CAD build for the part. Positions are in the model's coordinates, mm. Round coordinates to 2 decimals unless told otherwise and drop trailing zeros. Write each loop counter-clockwise with the first axis right and the second up, starting at its lowest first coordinate (ties: lowest second). Pieces come first, ordered by that corner, then holes. Notation, with made-up numbers: (-0.75, 43.5) - (18.25, 43.5) arc R15 cw to (18.25, 47.5) - close; hole circle Ø3 at (-20, 4.5). An arc over 180 degrees is marked (long way). Put each result on its own line as item: value. Start each with the question number.
Item 1: Cut at C-C (z = 3). Give the cut face in (x, y).
Item 2: Drill centre lines: line 1 (Z direction, x = 18, y = 3.9); line 2 (X direction, y = 1.05, z = 0); line 3 (X direction, y = 0.4, z = -0.75). Where is each one in solid material? Low to high. Write a range as from..to.
Item 3: Cut at B-B (y = 2.85). Count the separate pieces of the cut face and the enclosed holes in it, and give its area (3 significant figures).
Item 4: Cut at A-A (x = 18.25). Give the cut face in (y, z), and give its area (3 significant figures).
Item 5: Pin check, flat tip, straight feed: pin 1 Ø2 at (y, z) = (3.5, 1) entering from +X. Stop position of the tip, or through.
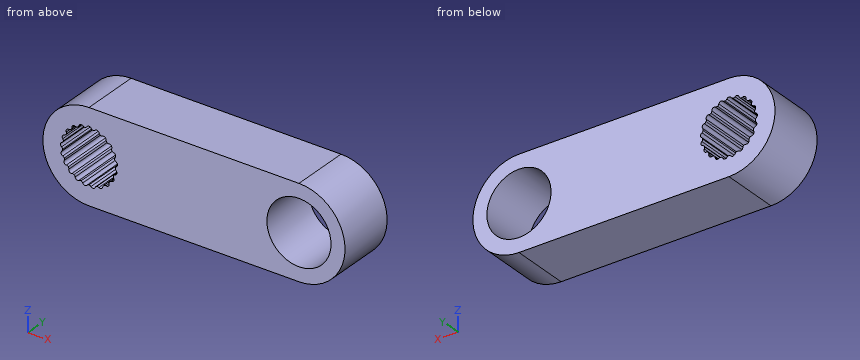
```python
from build123d import *

# Parameters (mm, degrees)
SKETCH1_R           = 3.95
BOSS_EXTRUDE1_DEPTH = 5
BOSS_EXTRUDE2_DEPTH = 5
SKETCH3_R           = 2.75
CUT_EXTRUDE1_DEPTH  = 5


with BuildPart() as part:
    # Sketch1 → Boss-Extrude1 (new body)
    with BuildSketch(Plane(origin=(0, 0, 0), x_dir=(1, 0, 0), z_dir=(0, 1, 0))):
        Circle(SKETCH1_R)
        with BuildLine():
            ThreePointArc((-0.166646614, 2.345141313), (-0.092401566, 2.286261662), (0, 2.2652595))
            ThreePointArc((0, 2.2652595), (0.092401566, 2.286261662), (0.166646614, 2.345141313))
            ThreePointArc((0.166646614, 2.345141313), (0.365153552, 2.422635524), (0.531999564, 2.290073216))
            ThreePointArc((0.531999564, 2.290073216), (0.585591031, 2.211925311), (0.667696959, 2.164620376))
            ThreePointArc((0.667696959, 2.164620376), (0.762183879, 2.157453631), (0.850485509, 2.191833312))
            ThreePointArc((0.850485509, 2.191833312), (1.063015161, 2.207373726), (1.183375246, 2.031522064))
            ThreePointArc((1.183375246, 2.031522064), (1.211551295, 1.941049689), (1.276066113, 1.871645232))
            ThreePointArc((1.276066113, 1.871645232), (1.364242809, 1.836946378), (1.458755034, 1.843771303))
            ThreePointArc((1.458755034, 1.843771303), (1.666423208, 1.795977086), (1.729602845, 1.592461261))
            ThreePointArc((1.729602845, 1.592461261), (1.72985991, 1.497703284), (1.771051193, 1.412366197))
            ThreePointArc((1.771051193, 1.412366197), (1.845082779, 1.353218377), (1.937407773, 1.331882123))
            ThreePointArc((1.937407773, 1.331882123), (2.121762239, 1.225), (2.12214764, 1.011903287))
            ThreePointArc((2.12214764, 1.011903287), (2.094462881, 0.92127937), (2.108670602, 0.827592226))
            ThreePointArc((2.108670602, 0.827592226), (2.161979047, 0.749250985), (2.243913329, 0.701649371))
            ThreePointArc((2.243913329, 0.701649371), (2.388573385, 0.545176288), (2.326130305, 0.341433266))
            ThreePointArc((2.326130305, 0.341433266), (2.272963633, 0.262995741), (2.258925375, 0.169283054))
            ThreePointArc((2.258925375, 0.169283054), (2.286773988, 0.078709355), (2.351037339, 0.009071994))
            ThreePointArc((2.351037339, 0.009071994), (2.443149303, -0.183088729), (2.323426084, -0.3593746))
            ThreePointArc((2.323426084, -0.3593746), (2.249501592, -0.418656214), (2.208464714, -0.504067659))
            ThreePointArc((2.208464714, -0.504067659), (2.208379026, -0.598825947), (2.249261363, -0.68431147))
            ThreePointArc((2.249261363, -0.68431147), (2.280640684, -0.89508551), (2.114275259, -1.028250455))
            ThreePointArc((2.114275259, -1.028250455), (2.026161462, -1.063108727), (1.961772273, -1.13262975))
            ThreePointArc((1.961772273, -1.13262975), (1.933759896, -1.223152935), (1.947628645, -1.316890857))
            ThreePointArc((1.947628645, -1.316890857), (1.915487132, -1.527550015), (1.717261799, -1.605761745))
            ThreePointArc((1.717261799, -1.605761745), (1.622787995, -1.613099364), (1.540767756, -1.660552716))
            ThreePointArc((1.540767756, -1.660552716), (1.487317713, -1.738797417), (1.472940575, -1.832458712))
            ThreePointArc((1.472940575, -1.832458712), (1.380134142, -2.024284997), (1.167662092, -2.040594058))
            ThreePointArc((1.167662092, -2.040594058), (1.075222693, -2.019759044), (0.982859262, -2.040928287))
            ThreePointArc((0.982859262, -2.040928287), (0.908720824, -2.099942118), (0.86737527, -2.185204569))
            ThreePointArc((0.86737527, -2.185204569), (0.722150177, -2.341153374), (0.514310485, -2.294110633))
            ThreePointArc((0.514310485, -2.294110633), (0.432119136, -2.246954269), (0.337619409, -2.239958423))
            ThreePointArc((0.337619409, -2.239958423), (0.249380102, -2.274497747), (0.184739867, -2.343785411))
            ThreePointArc((0.184739867, -2.343785411), (0, -2.45), (-0.184739867, -2.343785411))
            ThreePointArc((-0.184739867, -2.343785411), (-0.249380102, -2.274497747), (-0.337619409, -2.239958423))
            ThreePointArc((-0.337619409, -2.239958423), (-0.432119136, -2.246954269), (-0.514310485, -2.294110633))
            ThreePointArc((-0.514310485, -2.294110633), (-0.722150177, -2.341153374), (-0.86737527, -2.185204569))
            ThreePointArc((-0.86737527, -2.185204569), (-0.908720824, -2.099942118), (-0.982859262, -2.040928287))
            ThreePointArc((-0.982859262, -2.040928287), (-1.075222693, -2.019759044), (-1.167662092, -2.040594058))
            ThreePointArc((-1.167662092, -2.040594058), (-1.380134142, -2.024284997), (-1.472940575, -1.832458712))
            ThreePointArc((-1.472940575, -1.832458712), (-1.487317713, -1.738797417), (-1.540767756, -1.660552716))
            ThreePointArc((-1.540767756, -1.660552716), (-1.622787995, -1.613099364), (-1.717261799, -1.605761745))
            ThreePointArc((-1.717261799, -1.605761745), (-1.915487132, -1.527550015), (-1.947628645, -1.316890857))
            ThreePointArc((-1.947628645, -1.316890857), (-1.933759896, -1.223152935), (-1.961772273, -1.13262975))
            ThreePointArc((-1.961772273, -1.13262975), (-2.026161462, -1.063108727), (-2.114275259, -1.028250455))
            ThreePointArc((-2.114275259, -1.028250455), (-2.280640684, -0.89508551), (-2.249261363, -0.68431147))
            ThreePointArc((-2.249261363, -0.68431147), (-2.208379026, -0.598825947), (-2.208464714, -0.504067659))
            ThreePointArc((-2.208464714, -0.504067659), (-2.249501592, -0.418656214), (-2.323426084, -0.3593746))
            ThreePointArc((-2.323426084, -0.3593746), (-2.443149303, -0.183088729), (-2.351037339, 0.009071994))
            ThreePointArc((-2.351037339, 0.009071994), (-2.286773988, 0.078709355), (-2.258925375, 0.169283054))
            ThreePointArc((-2.258925375, 0.169283054), (-2.272963633, 0.262995741), (-2.326130305, 0.341433266))
            ThreePointArc((-2.326130305, 0.341433266), (-2.388573385, 0.545176288), (-2.243913329, 0.701649371))
            ThreePointArc((-2.243913329, 0.701649371), (-2.161979047, 0.749250985), (-2.108670602, 0.827592226))
            ThreePointArc((-2.108670602, 0.827592226), (-2.094462881, 0.92127937), (-2.12214764, 1.011903287))
            ThreePointArc((-2.12214764, 1.011903287), (-2.121762239, 1.225), (-1.937407773, 1.331882123))
            ThreePointArc((-1.937407773, 1.331882123), (-1.845082779, 1.353218377), (-1.771051193, 1.412366197))
            ThreePointArc((-1.771051193, 1.412366197), (-1.72985991, 1.497703284), (-1.729602845, 1.592461261))
            ThreePointArc((-1.729602845, 1.592461261), (-1.666423208, 1.795977086), (-1.458755034, 1.843771303))
            ThreePointArc((-1.458755034, 1.843771303), (-1.364242809, 1.836946378), (-1.276066113, 1.871645232))
            ThreePointArc((-1.276066113, 1.871645232), (-1.211551295, 1.941049689), (-1.183375246, 2.031522064))
            ThreePointArc((-1.183375246, 2.031522064), (-1.063015161, 2.207373726), (-0.850485509, 2.191833312))
            ThreePointArc((-0.850485509, 2.191833312), (-0.762183879, 2.157453631), (-0.667696959, 2.164620376))
            ThreePointArc((-0.667696959, 2.164620376), (-0.585591031, 2.211925311), (-0.531999564, 2.290073216))
            ThreePointArc((-0.531999564, 2.290073216), (-0.365153552, 2.422635524), (-0.166646614, 2.345141313))
        make_face(mode=Mode.SUBTRACT)
    extrude(amount=BOSS_EXTRUDE1_DEPTH)

    # Sketch2 → Boss-Extrude2 (add)
    with BuildSketch(Plane.XZ):
        with BuildLine():
            Line((0, 3.95), (18, 3.95))
            ThreePointArc((18, 3.95), (21.95, 0), (18, -3.95))
            Line((18, -3.95), (0, -3.95))
            ThreePointArc((0, -3.95), (3.95, 0), (0, 3.95))
        make_face()
    extrude(amount=-BOSS_EXTRUDE2_DEPTH)

    # Sketch3 → Cut-Extrude1 (cut)
    with BuildSketch(Plane(origin=(0, 5, 0), x_dir=(1, 0, 0), z_dir=(0, 1, 0))):
        with Locations((18, 0)):
            Circle(SKETCH3_R)
    extrude(amount=-CUT_EXTRUDE1_DEPTH, mode=Mode.SUBTRACT)


solid = part.part
```
Output values:
1. outline: (-2.57, 0) - (20.57, 0) - (20.57, 5) - (-2.57, 5) - close
2. line 1: -3.95..-2.75, 2.75..3.95
2. line 2: -3.95..-2.36, 2.36..15.25, 20.75..21.95
2. line 3: -3.88..-2.16, 2.16..15.35, 20.65..21.88
3. separate pieces: 1
3. enclosed holes: 2
3. area: 150 mm2
4. outline: (0, -3.94) - (5, -3.94) - (5, -2.74) - (0, -2.74) - close; (0, 2.74) - (5, 2.74) - (5, 3.94) - (0, 3.94) - close
4. area: 12.0 mm2
5. pin 1: x = 21.95
